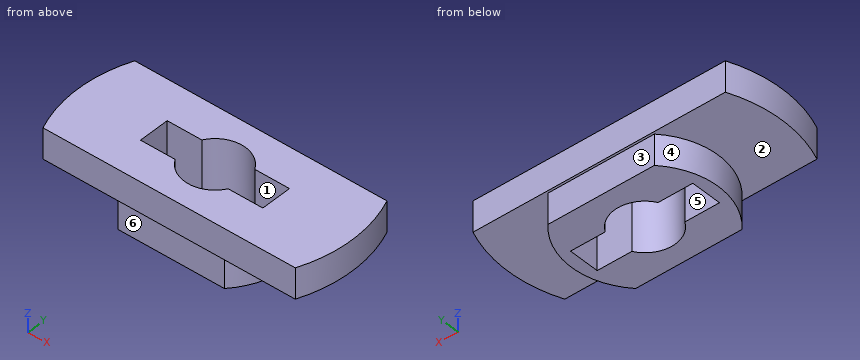
Autodesk Inventor part; units mm, degrees
ref_plane "YZ Plane" through (0, 0, 0) normal (1, 0, 0) x (0, 1, 0)
ref_plane "XZ Plane" through (0, 0, 0) normal (0, 1, 0) x (-1, 0, 0)
ref_plane "XY Plane" through (0, 0, 0) normal (0, 0, 1) x (1, 0, 0)
ref_plane "Work Plane1" through (0, 0, 0) normal (0, 0, 1) x (1, 0, 0)
sketch "Sketch1" plane through (0, 0, 0) normal (0, 0, 1) x (1, 0, 0)
  arc A0 (-3.5454, 3.44) -> (-3.5454, -3.44) centre (0, 0) ccw construction
  line L0 (-3.5454, 3.44) -> (-1.1656, 3.44) construction
  line L1 (-1.1656, 3.44) -> (-1.1656, 4.44) construction
  line L2 (-1.1656, 4.44) -> (-2.5, 4.44) construction
  line L3 (-2.5, 4.44) -> (-2.5, 5.44) construction
  line L4 (-2.5, 5.44) -> (2.5, 5.44) construction
  line L5 (2.5, 5.44) -> (2.5, 4.44) construction
  line L6 (2.5, 4.44) -> (1.1656, 4.44) construction
  line L7 (1.1656, 4.44) -> (1.1656, 3.44) construction
  line L8 (1.1656, 3.44) -> (3.5454, 3.44) construction
  arc A1 (3.5454, -3.44) -> (3.5454, 3.44) centre (0, 0) ccw construction
  line L9 (1.1656, -3.44) -> (3.5454, -3.44) construction
  line L10 (1.1656, -4.44) -> (1.1656, -3.44) construction
  line L11 (1.1656, -4.44) -> (2.5, -4.44) construction
  line L12 (2.5, -4.44) -> (2.5, -5.44) construction
  line L13 (2.5, -5.44) -> (-2.5, -5.44) construction
  line L14 (-2.5, -5.44) -> (-2.5, -4.44) construction
  line L15 (-1.1656, -4.44) -> (-2.5, -4.44) construction
  line L16 (-1.1656, -3.44) -> (-1.1656, -4.44) construction
  line L17 (-3.5454, -3.44) -> (-1.1656, -3.44) construction
  arc A2 (-11, 8.1244) -> (-11, -8.1244) centre (0, 0) ccw
  line L18 (-11, -8.1244) -> (-11, -24.74)
  line L19 (-11, -24.74) -> (11, -24.74)
  line L20 (11, -24.74) -> (11, -8.1244)
  arc A3 (11, -8.1244) -> (11, 8.1244) centre (0, 0) ccw
  line L21 (11, 24.74) -> (11, 8.1244)
  line L22 (-11, 24.74) -> (11, 24.74)
  line L23 (-11, 8.1244) -> (-11, 24.74)
  line L24 (-8.2517, 3.44) -> (8.2517, 3.44)
  line L25 (8.2517, 3.44) -> (8.2517, -3.44)
  line L26 (8.2517, -3.44) -> (-8.2517, -3.44)
  line L27 (-8.2517, -3.44) -> (-8.2517, 3.44)
  arc A4 (8.2517, -3.44) -> (8.2517, 3.44) centre (0, 0) ccw
  arc A5 (-8.2517, 3.44) -> (-8.2517, -3.44) centre (0, 0) ccw
  point P0 (0, 0)
extrude "Extrusion1" add sketch "Sketch1" along normal blind 2 contours L24 L25 L26 L27 | L27 A5 | A4 L25
sketch "Sketch2" plane through (0, 0, 0) normal (0, 0, -1) x (-1, 0, 0)
  line L0 (-8.2517, 3.44) -> (8.2517, 3.44) construction
  line L1 (8.2517, -3.44) -> (-8.2517, -3.44) construction
  line L2 (1.1656, -3.44) -> (3.5454, -3.44) construction
  line L3 (1.1656, -4.69) -> (1.1656, -3.44) construction
  line L4 (2.25, -4.69) -> (1.1656, -4.69) construction
  line L5 (2.25, -5.19) -> (2.25, -4.69) construction
  line L6 (-2.25, -5.19) -> (2.25, -5.19) construction
  line L7 (-2.25, -4.69) -> (-2.25, -5.19) construction
  line L8 (-1.1656, -4.69) -> (-2.25, -4.69) construction
  line L9 (-1.1656, -3.44) -> (-1.1656, -4.69) construction
  line L10 (-3.5454, -3.44) -> (-1.1656, -3.44) construction
  arc A0 (-3.5454, 3.44) -> (-3.5454, -3.44) centre (0, 0) ccw construction
  line L11 (-3.5454, 3.44) -> (-1.1656, 3.44) construction
  line L12 (-1.1656, 3.44) -> (-1.1656, 4.69) construction
  line L13 (-1.1656, 4.69) -> (-2.25, 4.69) construction
  line L14 (-2.25, 4.69) -> (-2.25, 5.19) construction
  line L15 (-2.25, 5.19) -> (2.25, 5.19) construction
  line L16 (2.25, 5.19) -> (2.25, 4.69) construction
  line L17 (2.25, 4.69) -> (1.1656, 4.69) construction
  line L18 (1.1656, 4.69) -> (1.1656, 3.44) construction
  line L19 (1.1656, 3.44) -> (3.5454, 3.44) construction
  arc A1 (3.5454, -3.44) -> (3.5454, 3.44) centre (0, 0) ccw construction
  circle A2 centre (0, 0) radius 6.94 construction
  circle A3 centre (0, 0) radius 4.79
  line L20 (-3.4814, 3.29) -> (3.4814, 3.29)
  line L21 (-3.4814, -3.29) -> (3.4814, -3.29)
  dimension "d3" = 0.15
  dimension "d4" = 0.15
  dimension "d5" = 0.15
extrude "Extrusion2" add sketch "Sketch2" along normal blind 2 contours A3 L21 L20
sketch "Sketch3" plane through (0, 0, -2) normal (0, 0, -1) x (-1, 0, 0)
  arc A0 (3.4814, -3.29) -> (3.4814, 3.29) centre (0, 0) ccw
  circle A1 centre (0, 0) radius 2
  line L0 (-4, -1) -> (4, -1)
  line L1 (4, -1) -> (4, 1)
  line L2 (4, 1) -> (-4, 1)
  line L3 (-4, 1) -> (-4, -1)
  line L4 (-4, -1) -> (4, 1) construction
  line L5 (4, -1) -> (-4, 1) construction
  dimension "d8" = 4
extrude "Extrusion3" cut sketch "Sketch3" against normal through all
properties part number "ECoG_holder_cap2"
Here's how the part is built. I have some questions about the finished solid (model axes, mm). Face numbers are marked on the shaded views. A direction names the side the tool comes from. Round coordinates to 2 decimals unless told otherwise and drop trailing zeros. Loops run counter-clockwise (first coordinate to the right, second up) from the corner with the lowest first, then second, coordinate; pieces in that order, holes last.
1. For P1, Ø1, axis at x = 0, z = -1.5, coming from the +Y side; P2, Ø4, axis at x = -1, y = -0.5, coming from the -Z side; P3, Ø2, axis at x = -1, z = -1.5, coming from the -Y side; P4, Ø1, axis at y = 1.5, z = -1.5, coming from the -X side, each with a flat end and sliding along its axis, tell me the tip position at first contact or that it passes through.
Answer list:
P1: stops at y = 3.29
P2: stops at z = -2
P3: stops at y = -3.29
P4: stops at x = -4.68
2. Which directions (+Z, -Z, +X, -X, +Y, -Y) give clear straight access to the entire face, cutting with the end or side of a thin tool? Please do the marked faces 4, 5 and 6.
Answer list:
face 4: -Z, -X
face 5: +Z, -Z
face 6: -Z, +X, -X, -Y
3. If we section it at C-C on x = 0.25: Write out the boundary of the cut face in (y, z).
Answer list:
outline: (-3.44, 0) - (-3.29, 0) - (-3.29, -2) - (-1.98, -2) - (-1.98, 2) - (-3.44, 2) - close; (1.98, -2) - (3.29, -2) - (3.29, 0) - (3.44, 0) - (3.44, 2) - (1.98, 2) - close
4. If we section it at B-B on y = -0.25: Write out the boundary of the cut face in (x, z).
Answer list:
outline: (-8.94, 0) - (-4.78, 0) - (-4.78, -2) - (-4, -2) - (-4, 2) - (-8.94, 2) - close; (4, -2) - (4.78, -2) - (4.78, 0) - (8.94, 0) - (8.94, 2) - (4, 2) - close
5. If we section it at A-A on z = 0.3: Write out the boundary of the cut face in (x, y).
Answer list:
outline: (-8.25, -3.44) - (8.25, -3.44) arc R8.94 ccw to (8.25, 3.44) - (-8.25, 3.44) arc R8.94 ccw to start; hole (-4, -1) - (-1.73, -1) arc R2 ccw to (1.73, -1) - (4, -1) - (4, 1) - (1.73, 1) arc R2 ccw to (-1.73, 1) - (-4, 1) - close
6. If I drill on line 1 along Y through (x, z) = (2.5, 1.65); line 2 along X through (y, z) = (-0.25, 0.4); line 3 along Y through (x, z) = (2, -0.4), over which ranges is the centre line in solid material (lowest first)?
Answer list:
line 1: y = -3.44 to -1, 1 to 3.44
line 2: x = -8.94 to -4, 4 to 8.94
line 3: y = -3.29 to -1, 1 to 3.29
7. If we section it at D-D on y = -2.75: Write out the boundary of the cut face in (x, z).
Answer list:
outline: (-8.51, 0) - (-3.92, 0) - (-3.92, -2) - (3.92, -2) - (3.92, 0) - (8.51, 0) - (8.51, 2) - (-8.51, 2) - close
8. We'd pull the mould along Y, two halves only. Please class the marked faces 1, 2 and 3: +Y half, -Y half, draft (parallel to the pull), parting line (faces both ways), or undercut.
Answer list:
face 1: undercut
face 2: draft
face 3: +Y half
